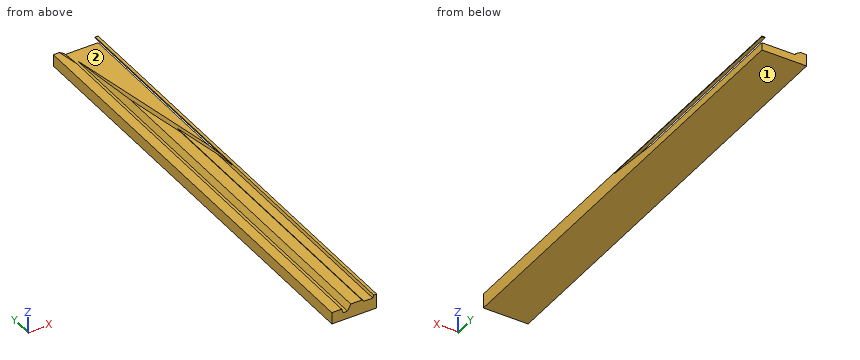
```python
from build123d import *

# Parameters (mm, degrees)
F0_W          = 250
F0_H          = 88
F1_DEPTH      = 2500
F3_DEPTH      = 2500.001
F7_DEPTH      = 2492.408814
F7_DEPTH_BACK = 25


with BuildPart() as f1:
    # F0 (on Front) → F1 (new body)
    with BuildSketch(Plane.XZ):
        with Locations((125, 44)):
            Rectangle(F0_W, F0_H)
    extrude(amount=F1_DEPTH)

    # F2 (on Front) → F3 (cut, through all)
    with BuildSketch(Plane.XZ):
        Polygon((-6.027462, 133.504351), (-6.027462, 65.639846), (54.952722, 65.639846), (63.961156, 42.079318), (87.521672, 42.079318), (105.538554, 76.727152), (167.904645, 76.727152), (178.991958, 65.639846), (228.191867, 65.639846), (233.735517, 80.884889), (266.304493, 80.884889), (266.304493, 133.504351), align=None)
    extrude(amount=F3_DEPTH, mode=Mode.SUBTRACT)

    # F6 (on face) → F7 (cut, two sides)
    with BuildSketch(Plane(origin=(2.261527, -12.825755, 0), x_dir=(0.984808, 0.173648, 0), z_dir=(0.173648, -0.984808, 0))) as f7_sk:
        Polygon((13.848773, 76.727152), (73.860581, 42.079318), (295.860581, 42.079318), (295.860581, 76.727152), align=None)
    extrude(amount=F7_DEPTH, mode=Mode.SUBTRACT)
    extrude(f7_sk.sketch, amount=-F7_DEPTH_BACK, mode=Mode.SUBTRACT)


solid = f1.part
```
Source: CAD feature listing. Evaluate the final solid. Frame: model axes, mm. Face numbers are marked on the shaded views. Round coordinates to 2 decimals unless told otherwise and drop trailing zeros. Loops run counter-clockwise (first coordinate to the right, second up) from the corner with the lowest first, then second, coordinate; pieces in that order, holes last. Notation, with made-up numbers: M -31.5,-7 L -20.5,-7 A23 cw -20.5,18 Z; hole C 67.5,72.5 d2. An arc over 180 degrees is marked long. Use a Markdown table: item, result. Add a question column.
1. Cut plane A-A, the plane y = -1191.5. Output: boundary loops of the cut face in (x, z), and give its area (3 significant figures).
2. Cut plane D-D, the plane y = -542. Output: boundary loops of the cut face in (x, z).
3. Cut plane B-B, the plane y = -1532.5. Output: boundary loops of the cut face in (x, z), and give its area (3 significant figures).
4. Ray query, line 1 along Z through (x, y) = (219, -1857); line 2 along Z through (x, y) = (136.5, -1886); line 3 along X through (y, z) = (-1494, 51.5). Return the intervals inside material, ascending. Write a range as [from, to].
5. Pull-direction query (X, two-part tool) for the marked faces 1 and 2; classes: +X half, -X half, draft (parallel to the pull), parting line (faces both ways), or undercut.
6. Cut plane C-C, the plane x = 140.5. Output: boundary loops of the cut face in (y, z), and give its area (3 significant figures).
7. Contact query for flat-ended pins moving along their axis: pin 1 (3 mm diameter, centred on x = 174.5, y = -1270.5, fed in from +Z); pin 2 (24.5 mm diameter, centred on x = 199, y = -1322.5, fed in from +Z). Output: stop coordinate, or through.
Solution:
| question | item | result |
|---|---|---|
| 1 | outline | M 0,0 L 250,0 L 250,62.03 L 230.84,72.93 L 228.19,65.64 L 178.99,65.64 L 167.9,76.73 L 105.54,76.73 L 87.52,42.08 L 63.96,42.08 L 54.95,65.64 L 0,65.64 Z; M 232.22,76.73 L 250,76.73 L 250,80.88 L 233.74,80.88 Z |
| 1 | area | 16,500 mm2 |
| 2 | outline | M 0,0 L 250,0 L 250,42.08 L 170.57,42.08 L 109.63,76.73 L 105.54,76.73 L 87.52,42.08 L 63.96,42.08 L 54.95,65.64 L 0,65.64 Z; M 232.22,76.73 L 250,76.73 L 250,80.88 L 233.74,80.88 Z |
| 3 | outline | M 0,0 L 250,0 L 250,80.88 L 233.74,80.88 L 228.19,65.64 L 178.99,65.64 L 167.9,76.73 L 105.54,76.73 L 87.52,42.08 L 63.96,42.08 L 54.95,65.64 L 0,65.64 Z |
| 3 | area | 16,700 mm2 |
| 4 | line 1 | z = [0, 65.64] |
| 4 | line 2 | z = [0, 76.73] |
| 4 | line 3 | x = [0, 60.36], [92.42, 250] |
| 5 | face 1 | draft |
| 5 | face 2 | undercut |
| 6 | outline | M -2500,0 L 0,0 L 0,42.08 L -371.47,42.08 L -717.06,76.73 L -2500,76.73 Z |
| 6 | area | 173,000 mm2 |
| 7 | pin 1 | stops at z = 71.63 |
| 7 | pin 2 | stops at z = 65.64 |
